The listing builds one solid part. Answer for the finished solid, in the listing's coordinates (mm). A direction names the side the tool comes from. Coordinates: 2 decimals unless noted, no trailing zeros. Write each loop counter-clockwise with the first axis right and the second up, starting at its lowest first coordinate (ties: lowest second). Pieces come first, ordered by that corner, then holes.
(1) The part is cut by section A-A on x = 0. Determine the outline of the cut face in (y, z), plus the area to 3 significant figures.
(2) Which of the six approach directions +Z, -Z, +X, -X, +Y, -Y give full straight-line access (tool end or side, diameter ignored) to faces 1 (the cylindrical face through (-5, -8, 0)), 2 (the flat face through (0, -5, -23.748)), 3 (the flat face through (10, -5, -19))?
(3) Straight lines are drawn through the part: line 1 (Z direction, x = 0, y = -9.5); line 2 (Y direction, x = 11, z = 0); line 3 (Y direction, x = -0.5, z = -6). For each, find the intervals that lie inside material, in ascending order.
(4) Given P1, Ø8, axis at y = -3, z = -9, coming from the +X side; P2, Ø10, axis at x = 5.5, z = -8.5, coming from the -Y side; P3, Ø8, axis at y = -5, z = -20, coming from the +X side, each flat-ended and moving along its own axis, determine where each tip first touches the part or whether it passes through.
(5) For a pull along X with two mould halves and no side action, classify faces 4 (the flat face through (2.5, -8, -10)), 5 (the flat face through (-10, -5, -19)), 6 (the flat face through (3.5, -10, -3.1)) as +X half, -X half, draft (parallel to the pull), parting line (faces both ways), or undercut.
(6) The part is cut by section C-C on y = -4.5. Determine the outline of the cut face in (x, z).
(7) The part is cut by section D-D on x = -8. Determine the outline of the cut face in (y, z).
(8) The part is cut by section B-B on z = -18.5. Determine the outline of the cut face in (x, y), plus the area to 3 significant figures.
from build123d import *

# Parameters (mm, degrees)
F1_DEPTH = 10
F3_DEPTH = 4
F4_R     = 3.4
F5_DEPTH = 8


# Not quite as in the source:
# - a feature of the source that left no trace in its solid (it failed there, or was rolled back) is left out
# - a pattern or mirror of a feature is missing from the dataset's text; its kind, count and spacing are read off the source's solid


with BuildPart() as f1:
    # F0 (on Front) → F1 (new body)
    with BuildSketch(Plane.XZ):
        with BuildLine():
            ThreePointArc((10, -13.7477270849), (15.1492574075, -7.7136243103), (17, 0))
            ThreePointArc((17, 0), (-7.7136243103, 15.1492574075), (-10, -13.7477270849))
            ThreePointArc((-10, -13.7477270849), (0, -17), (10, -13.7477270849))
        make_face()
        with BuildLine():
            ThreePointArc((10, -13.7477270849), (0, -17), (-10, -13.7477270849))
            Line((-10, -13.7477270849), (-10, -23.7477270849))
            Line((-10, -23.7477270849), (10, -23.7477270849))
            Line((10, -23.7477270849), (10, -13.7477270849))
        make_face()
    extrude(amount=F1_DEPTH)

    # F2 (on face) → F3 (cut)
    with BuildSketch(Plane.XZ.offset(10)):
        with BuildLine():
            Line((-2.5, 4.3301270189), (-2.5, 14.7901994577))
            ThreePointArc((-2.5, 14.7901994577), (-15, 0), (-2.5, -14.7901994577))
            Line((-2.5, -14.7901994577), (-2.5, -4.3301270189))
            ThreePointArc((-2.5, -4.3301270189), (-5, 0), (-2.5, 4.3301270189))
        make_face()
    f3 = extrude(amount=-F3_DEPTH, mode=Mode.SUBTRACT)

    # F3_copies: F3 across plane
    add(f3.mirror(Plane(origin=(0, 0, 0), x_dir=(0, 0, 1), z_dir=(1, 0, 0))), mode=Mode.SUBTRACT)

    # F4 (on face) → F5 (join)
    with BuildSketch(Plane.XZ.offset(10)):
        Circle(F4_R)
    extrude(amount=F5_DEPTH)


solid = f1.part
Model answer:
1. outline: (-18, -3.4) - (-10, -3.4) - (-10, -23.75) - (0, -23.75) - (0, 17) - (-10, 17) - (-10, 3.4) - (-18, 3.4) - close
1. area: 462 mm2
2. face 1: -Y
2. face 2: -Z, +X, -X, +Y, -Y
2. face 3: -Z, +X, +Y, -Y
3. line 1: z = -23.75 to 17
3. line 2: y = -6 to 0
3. line 3: y = -10 to 0
4. P1: stops at x = 16.25
4. P2: stops at y = -10
4. P3: stops at x = 10
5. face 4: undercut
5. face 5: -X half
5. face 6: draft
6. outline: (-10, -23.75) - (10, -23.75) - (10, -13.75) arc R17 ccw (long way) to (-10, -13.75) - close
7. outline: (-10, -23.75) - (0, -23.75) - (0, 15) - (-10, 15) - (-10, 12.69) - (-6, 12.69) - (-6, -12.69) - (-10, -12.69) - close
8. outline: (-10, -10) - (10, -10) - (10, 0) - (-10, 0) - close
8. area: 200 mm2
